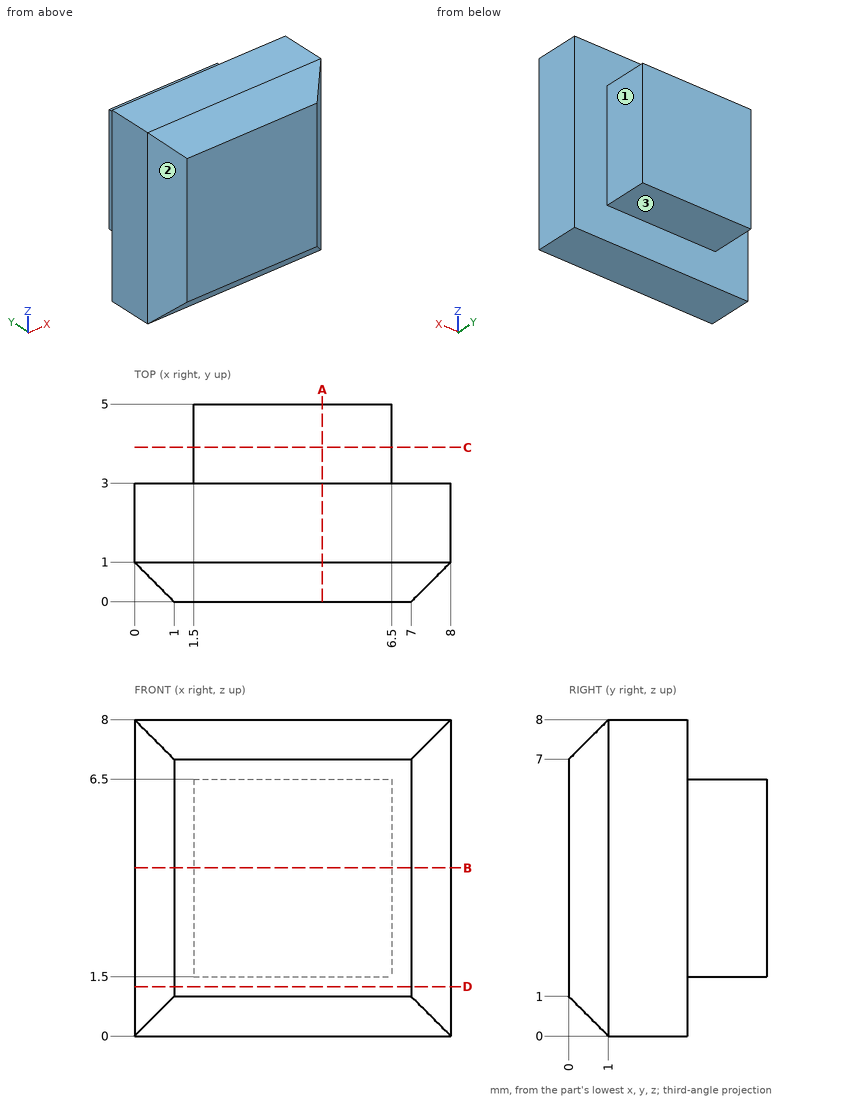
Job drawing, mm, ordinate dimensions from the low corner. One solid piece. A direction names the side the tool comes from. Coordinates: 2 decimals unless noted, no trailing zeros. Order: outer loops, then holes, each group sorted by start corner. A loop starts at its lowest first (then second) coordinate and runs counter-clockwise, first axis right, second up. Notation, with made-up numbers: (37.5, 4) -> (80.5, 4) arc R35 cw to (80.5, 37) -> close; hole circle Ø1 at (-20, 89.25). An arc over 180 degrees is marked (long way). Answer in a Markdown table with one row per item. Add a question column.
Q1. Band-saw the part on A-A, the plane x = 4.75. List the corners of the cut face in (y, z).
Q2. Drop flat-ended pins along their axis: pin 1 (1.6 mm diameter, centred on x = 4.5, y = 4, fed in from -Z); pin 2 (1 mm diameter, centred on y = 4, z = 4, fed in from -X); pin 3 (1 mm diameter, centred on x = 3.5, y = 4.5, fed in from +Z). Give the stop position or say it passes through.
Q3. Which spindle directions (+Z, -Z, +X, -X, +Y, -Y) get a long thin tool onto all of the face, cutting with end or side? Do the marked faces 1, 2 and 3. Say none if no direction does.
Q4. Wall check: line 1 along Z through (x, y) = (2.5, 4.35); line 2 along Y through (x, z) = (1.25, 4.25). Give the ranges that are in metal, low to high. Write a range as [from, to].
Q5. Band-saw the part on D-D, the plane z = 1.25. List the corners of the cut face in (x, y), then the cut area to 3 significant figures.
Q6. Band-saw the part on B-B, the plane z = 4.25. List the corners of the cut face in (x, y).
Q7. Band-saw the part on C-C, the plane y = 3.9. List the corners of the cut face in (x, z), then the cut area to 3 significant figures.
Answers follow:
| question | item | result |
|---|---|---|
| 1 | outline | (0, 1) -> (1, 0) -> (3, 0) -> (3, 1.5) -> (5, 1.5) -> (5, 6.5) -> (3, 6.5) -> (3, 8) -> (1, 8) -> (0, 7) -> close |
| 2 | pin 1 | z = 1.5 |
| 2 | pin 2 | x = 1.5 |
| 2 | pin 3 | z = 6.5 |
| 3 | face 1 | +Z, -Z, +X, +Y |
| 3 | face 2 | +Z, -Z, -X, -Y |
| 3 | face 3 | -Z, +X, -X, +Y |
| 4 | line 1 | [1.5, 6.5] |
| 4 | line 2 | [0, 3] |
| 5 | outline | (0, 1) -> (1, 0) -> (7, 0) -> (8, 1) -> (8, 3) -> (0, 3) -> close |
| 5 | area | 23.0 mm^2 |
| 6 | outline | (0, 1) -> (1, 0) -> (7, 0) -> (8, 1) -> (8, 3) -> (6.5, 3) -> (6.5, 5) -> (1.5, 5) -> (1.5, 3) -> (0, 3) -> close |
| 7 | outline | (1.5, 1.5) -> (6.5, 1.5) -> (6.5, 6.5) -> (1.5, 6.5) -> close |
| 7 | area | 25.0 mm^2 |
